Build history of the part. All positions in model axes, mm. A direction names the side the tool comes from. Round coordinates to 2 decimals unless told otherwise and drop trailing zeros. Write each loop counter-clockwise with the first axis right and the second up, starting at its lowest first coordinate (ties: lowest second). Pieces come first, ordered by that corner, then holes.
1) Saw through at B-B (y = -8.5). Write the cut outline in (x, z), plus the area to 3 significant figures.
2) Flat gauge pins, fed straight in: pin 1 (8 mm diameter, centred on x = 4, y = -4.5, fed in from -Z); pin 2 (3 mm diameter, centred on x = 5, z = -4.5, fed in from +Y). Where does each tip first touch, or does it go through?
3) Saw through at C-C (x = -8). Write the cut outline in (y, z).
4) Saw through at D-D (y = 7.75). Write the cut outline in (x, z), plus the area to 3 significant figures.
5) Wall check: probe 1 along X at (y, z) = (-7.75, -6.75); probe 2 along Z at (x, y) = (0, -0.5). Give the ranges that are in metal, low to high.
6) Which spindle directions (+Z, -Z, +X, -X, +Y, -Y) get a long thin tool onto all of the face, cutting with end or side? Do faces 1 (the flat face through (-7.278, -9, -5)), 2 (the flat face through (-6.86, 9, -5)), 3 (the flat face through (9, 7.394, -5)), 4 (the flat face through (-8, 7.289, -5)). Say none if no direction does.
7) Pull direction X, two halves, no side cores. Call faces 5 (the flat face through (-2, 10, 1)), 6 (the flat face through (7.375, 9, -5)), 7 (the flat face through (-10, -9, -5)), 8 (the flat face through (10, 2, 1)): +X half, -X half, draft (parallel to the pull), parting line (faces both ways), or undercut.
8) Saw through at A-A (z = -1.5). Write the cut outline in (x, y).
from build123d import *

# Parameters (mm, degrees)
F0_W     = 20
F0_H     = 20
F1_DEPTH = 5
F2_W     = 2.721561
F2_H     = 2.947924
F2_W_2   = 2.833921
F2_H_2   = 2.843244
F2_W_3   = 2.62458
F2_H_3   = 2.606365
F2_W_4   = 3.140243
F2_H_4   = 2.711044
F3_DEPTH = 10


with BuildPart() as f1:
    # F0 (on Top) → F1 (new body)
    with BuildSketch(Plane.XY):
        Rectangle(F0_W, F0_H)
    extrude(amount=F1_DEPTH)

    # F2 (on face) → F3 (join)
    with BuildSketch(Plane(origin=(0, 0, 0), x_dir=(1, 0, 0), z_dir=(0, 0, -1))):
        with Locations((-8.639219, 8.526038)):
            Rectangle(F2_W, F2_H)
        with Locations((8.583039, 8.578378)):
            Rectangle(F2_W_2, F2_H_2)
        with Locations((8.68771, -8.696817)):
            Rectangle(F2_W_3, F2_H_3)
        with Locations((-8.429879, -8.644478)):
            Rectangle(F2_W_4, F2_H_4)
    extrude(amount=F3_DEPTH)


solid = f1.part
Evaluation:
1. outline: (-10, -10) - (-7.28, -10) - (-7.28, 0) - (7.17, 0) - (7.17, -10) - (10, -10) - (10, 5) - (-10, 5) - close
1. area: 156 mm2
2. pin 1: stops at z = 0
2. pin 2: passes through
3. outline: (-10, -10) - (-7.05, -10) - (-7.05, 0) - (7.29, 0) - (7.29, -10) - (10, -10) - (10, 5) - (-10, 5) - close
4. outline: (-10, -10) - (-6.86, -10) - (-6.86, 0) - (7.38, 0) - (7.38, -10) - (10, -10) - (10, 5) - (-10, 5) - close
4. area: 158 mm2
5. probe 1: x = -10 to -7.28, 7.17 to 10
5. probe 2: z = 0 to 5
6. face 1: -Z, -Y
6. face 2: -Z, +Y, -Y
6. face 3: -Z, +X
6. face 4: -Z, +X, -X
7. face 5: draft
7. face 6: undercut
7. face 7: -X half
7. face 8: +X half
8. outline: (-10, -10) - (-7.28, -10) - (-7.28, -7.05) - (-10, -7.05) - close; (-10, 7.29) - (-6.86, 7.29) - (-6.86, 10) - (-10, 10) - close; (7.17, -10) - (10, -10) - (10, -7.16) - (7.17, -7.16) - close; (7.38, 7.39) - (10, 7.39) - (10, 10) - (7.38, 10) - close
